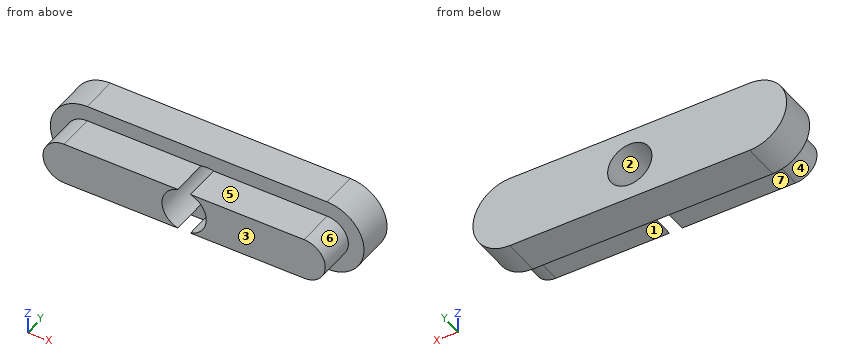
```python
from build123d import *

# Parameters (mm, degrees)
BOSS_EXTRUDE1_DEPTH = 2
BOSS_EXTRUDE2_DEPTH = 2
SKETCH3_R           = 1.2
CUT_EXTRUDE1_DEPTH  = 5


with BuildPart() as part:
    # Sketch1 → Boss-Extrude1 (new body)
    with BuildSketch(Plane(origin=(0, 0, 0), x_dir=(1, 0, 0), z_dir=(0, 1, 0))):
        with BuildLine():
            Line((-6.5, 2), (6.5, 2))
            ThreePointArc((6.5, 2), (8.5, 0), (6.5, -2))
            Line((6.5, -2), (-6.5, -2))
            ThreePointArc((-6.5, -2), (-8.5, 0), (-6.5, 2))
        make_face()
    extrude(amount=BOSS_EXTRUDE1_DEPTH)

    # Sketch2 → Boss-Extrude2 (add)
    with BuildSketch(Plane.XZ):
        with BuildLine():
            Line((-6.5, 1.15), (6.5, 1.15))
            ThreePointArc((6.5, 1.15), (7.65, 0), (6.5, -1.15))
            Line((6.5, -1.15), (-6.5, -1.15))
            ThreePointArc((-6.5, -1.15), (-7.65, 0), (-6.5, 1.15))
        make_face()
    extrude(amount=BOSS_EXTRUDE2_DEPTH)

    # Sketch3 → Cut-Extrude1 (cut, through all)
    with BuildSketch(Plane.XZ.offset(2)):
        Circle(SKETCH3_R)
    extrude(amount=-CUT_EXTRUDE1_DEPTH, mode=Mode.SUBTRACT)


solid = part.part
```
Geometry check sheet. Reference: the model listing, model coordinates, mm. Face numbers are marked on the shaded views. A direction names the side the tool comes from. Coordinates: 2 decimals unless noted, no trailing zeros. Write each loop counter-clockwise with the first axis right and the second up, starting at its lowest first coordinate (ties: lowest second). Pieces come first, ordered by that corner, then holes. Notation, with made-up numbers: M 28.5,24 L 40.5,24 A33 cw 40.5,53 Z; hole C 14,45.25 d10. An arc over 180 degrees is marked long. Answer as a JSON object with one key per item and string values.
1. Section check B-B, the plane y = -0.4. Enter the section's corners in (x, z), plus the area to 3 significant figures.
Answers below:
{"outline": "M -6.5,-1.15 L -0.34,-1.15 A1.2 cw -0.34,1.15 L -6.5,1.15 A1.15 ccw Z; M 0.34,-1.15 L 6.5,-1.15 A1.15 ccw 6.5,1.15 L 0.34,1.15 A1.2 cw Z", "area": "29.6 mm²"}
2. Scan lines: L1, parallel to X at y = 0.4, z = 0; L2, parallel to Z at x = 0, y = 0.7; L3, parallel to X at y = -1, z = 0. Record each from-to range of solid material in increasing order.
Answers below:
{"L1": "x = -8.5 to -1.2, 1.2 to 8.5", "L2": "z = -2 to -1.2, 1.2 to 2", "L3": "x = -7.65 to -1.2, 1.2 to 7.65"}
3. Tool access check on the marked faces 4, 5, 6 and 7. Record the directions out of +Z, -Z, +X, -X, +Y, -Y that give a thin tool (end or side, any length) a straight path to the whole face; none if there is none.
Answers below:
{"face 4": "-X, -Y", "face 5": "+Z, +X, -X, -Y", "face 6": "+X, -Y", "face 7": "-Z, +X, -X, -Y"}
4. Section check A-A, the plane x = 0. Enter the section's corners in (y, z).
Answers below:
{"outline": "M 0,-2 L 2,-2 L 2,-1.2 L 0,-1.2 Z; M 0,1.2 L 2,1.2 L 2,2 L 0,2 Z"}
5. Section check C-C, the plane z = 0. Enter the section's corners in (x, y), plus the area to 3 significant figures.
Answers below:
{"outline": "M -8.5,0 L -7.65,0 L -7.65,-2 L -1.2,-2 L -1.2,2 L -8.5,2 Z; M 1.2,-2 L 7.65,-2 L 7.65,0 L 8.5,0 L 8.5,2 L 1.2,2 Z", "area": "55.0 mm²"}
6. Go/stop test with flat-tipped pins: pin 1 Ø1.6 at (x, y) = (-4, -1) entering from -Z; pin 2 Ø1 at (x, y) = (0.5, -1) entering from -Z; pin 3 Ø1.5 at (y, z) = (-1.5, 0.5) entering from +X. Record where each tip stops, or that it passes through.
Answers below:
{"pin 1": "stops at z = -1.15", "pin 2": "stops at z = -1.15", "pin 3": "stops at x = 7.65"}
7. Draft check along Z on the marked faces 1, 2 and 3. Enter one of: released by +Z, released by -Z, zero draft, split by the parting line, or undercut.
Answers below:
{"face 1": "released by -Z", "face 2": "undercut", "face 3": "zero draft"}
8. Section check D-D, the plane y = 1.85. Enter the section's corners in (x, z).
Answers below:
{"outline": "M -6.5,-2 L 6.5,-2 A2 ccw 6.5,2 L -6.5,2 A2 ccw Z; hole C 0,0 d2.4"}
